CAD build for the part. Positions are in the model's coordinates, mm. Face numbers are marked on the shaded views. A direction names the side the tool comes from. Give positions to 0.01 mm unless a question says otherwise; leave off trailing zeros. Write each loop counter-clockwise with the first axis right and the second up, starting at its lowest first coordinate (ties: lowest second). Pieces come first, ordered by that corner, then holes. Notation, with made-up numbers: M -37.5,-1.75 L -1.5,-1.75 A11 ccw -1.5,2.25 Z; hole C 65,-17.75 d6. An arc over 180 degrees is marked long. One line per question, with ' | ' between items. Start each with the question number.
1. Cut at A-A, the plane x = 7. Write the cut outline in (y, z), then the cut area to 3 significant figures.
2. Wall check: L1, parallel to Y at x = 8.25, z = -1.25; L2, parallel to Z at x = -7, y = 0.4; L3, parallel to Y at x = -0.5, z = -3. Give the ranges that are in metal, low to high.
3. Cut at B-B, the plane y = 1.25. Write the cut outline in (x, z), then the cut area to 3 significant figures.
4. Flat gauge pins, fed straight in: pin 1 (1 mm diameter, centred on y = 5.5, z = 3.5, fed in from +X); pin 2 (5 mm diameter, centred on y = 8, z = -2, fed in from -X); pin 3 (1.5 mm diameter, centred on x = 3, y = 2, fed in from -Z); pin 4 (1.6 mm diameter, centred on x = -7, z = 0, fed in from +Y). Where does each tip first touch, or does it go through?
5. Which spindle directions (+Z, -Z, +X, -X, +Y, -Y) get a long thin tool onto all of the face, cutting with end or side? Do the marked faces 1 and 2. Say none if no direction does.
```python
from build123d import *

# Parameters (mm, degrees)
BOSS_EXTRUDE1_DEPTH = 1
SKETCH2_R           = 5.5
BOSS_EXTRUDE2_DEPTH = 8
FILLET1_R           = 5


with BuildPart() as part:
    # Sketch1 → Boss-Extrude1 (new body)
    with BuildSketch(Plane(origin=(0, 0, 0), x_dir=(1, 0, 0), z_dir=(0, 1, 0))):
        with BuildLine():
            ThreePointArc((-8, 0), (-7, 1), (-6, 0))
            ThreePointArc((-6, 0), (-5.905505906, 1.060660172), (-5.625, 2.087911636))
            ThreePointArc((-5.625, 2.087911636), (-6.926553741, 2.498920897), (-8.25, 2.165063509))
            ThreePointArc((-8.25, 2.165063509), (-9.165063509, 1.25), (-9.5, 0))
            Line((-9.5, 0), (-8, 0))
        make_face()
        with BuildLine():
            ThreePointArc((-5.625, -2.087911636), (-5.905505906, -1.060660172), (-6, 0))
            ThreePointArc((-6, 0), (-7, -1), (-8, 0))
            Line((-8, 0), (-9.5, 0))
            ThreePointArc((-9.5, 0), (-9.165063509, -1.25), (-8.25, -2.165063509))
            ThreePointArc((-8.25, -2.165063509), (-6.926553741, -2.498920897), (-5.625, -2.087911636))
        make_face()
        with BuildLine():
            ThreePointArc((-5.625, 2.087911636), (-5.905505906, 1.060660172), (-6, 0))
            Line((-6, 0), (-4.5, 0))
            ThreePointArc((-4.5, 0), (-4.799147892, 1.185854123), (-5.625, 2.087911636))
        make_face()
        with BuildLine():
            Line((-4.5, 0), (-6, 0))
            ThreePointArc((-6, 0), (-5.905505906, -1.060660172), (-5.625, -2.087911636))
            ThreePointArc((-5.625, -2.087911636), (-4.799147892, -1.185854123), (-4.5, 0))
        make_face()
        with BuildLine():
            ThreePointArc((-8.25, 2.165063509), (-6.926553741, 2.498920897), (-5.625, 2.087911636))
            ThreePointArc((-5.625, 2.087911636), (-4.58398805, 3.871311606), (-3, 5.196152423))
            Line((-3, 5.196152423), (-8.25, 2.165063509))
        make_face()
        with BuildLine():
            ThreePointArc((-3, -5.196152423), (-4.58398805, -3.871311606), (-5.625, -2.087911636))
            ThreePointArc((-5.625, -2.087911636), (-6.926553741, -2.498920897), (-8.25, -2.165063509))
            Line((-8.25, -2.165063509), (-3, -5.196152423))
        make_face()
        with BuildLine():
            Line((4.5, 0), (-4.5, 0))
            ThreePointArc((-4.5, 0), (-4.799147892, -1.185854123), (-5.625, -2.087911636))
            ThreePointArc((-5.625, -2.087911636), (-4.58398805, -3.871311606), (-3, -5.196152423))
            Line((-3, -5.196152423), (3, -5.196152423))
            ThreePointArc((3, -5.196152423), (4.58398805, -3.871311606), (5.625, -2.087911636))
            ThreePointArc((5.625, -2.087911636), (4.799147892, -1.185854123), (4.5, 0))
        make_face()
        with BuildLine():
            ThreePointArc((-5.625, 2.087911636), (-4.799147892, 1.185854123), (-4.5, 0))
            Line((-4.5, 0), (4.5, 0))
            ThreePointArc((4.5, 0), (4.799147892, 1.185854123), (5.625, 2.087911636))
            ThreePointArc((5.625, 2.087911636), (4.58398805, 3.871311606), (3, 5.196152423))
            ThreePointArc((3, 5.196152423), (0, 6), (-3, 5.196152423))
            ThreePointArc((-3, 5.196152423), (-4.58398805, 3.871311606), (-5.625, 2.087911636))
        make_face()
        with BuildLine():
            Line((3, -5.196152423), (-3, -5.196152423))
            ThreePointArc((-3, -5.196152423), (0, -6), (3, -5.196152423))
        make_face()
        with BuildLine():
            ThreePointArc((3, 5.196152423), (4.58398805, 3.871311606), (5.625, 2.087911636))
            ThreePointArc((5.625, 2.087911636), (6.926553741, 2.498920897), (8.25, 2.165063509))
            Line((8.25, 2.165063509), (3, 5.196152423))
        make_face()
        with BuildLine():
            ThreePointArc((8.25, -2.165063509), (6.926553741, -2.498920897), (5.625, -2.087911636))
            ThreePointArc((5.625, -2.087911636), (4.58398805, -3.871311606), (3, -5.196152423))
            Line((3, -5.196152423), (8.25, -2.165063509))
        make_face()
        with BuildLine():
            ThreePointArc((5.625, 2.087911636), (4.799147892, 1.185854123), (4.5, 0))
            Line((4.5, 0), (6, 0))
            ThreePointArc((6, 0), (5.905505906, 1.060660172), (5.625, 2.087911636))
        make_face()
        with BuildLine():
            Line((6, 0), (4.5, 0))
            ThreePointArc((4.5, 0), (4.799147892, -1.185854123), (5.625, -2.087911636))
            ThreePointArc((5.625, -2.087911636), (5.905505906, -1.060660172), (6, 0))
        make_face()
        with BuildLine():
            ThreePointArc((8, 0), (7, -1), (6, 0))
            ThreePointArc((6, 0), (5.905505906, -1.060660172), (5.625, -2.087911636))
            ThreePointArc((5.625, -2.087911636), (6.926553741, -2.498920897), (8.25, -2.165063509))
            Line((8.25, -2.165063509), (8.25, 0))
            Line((8.25, 0), (8, 0))
        make_face()
        with BuildLine():
            ThreePointArc((5.625, 2.087911636), (5.905505906, 1.060660172), (6, 0))
            ThreePointArc((6, 0), (7, 1), (8, 0))
            Line((8, 0), (8.25, 0))
            Line((8.25, 0), (8.25, 2.165063509))
            ThreePointArc((8.25, 2.165063509), (6.926553741, 2.498920897), (5.625, 2.087911636))
        make_face()
        with BuildLine():
            ThreePointArc((9.5, 0), (9.165063509, 1.25), (8.25, 2.165063509))
            Line((8.25, 2.165063509), (8.25, 0))
            Line((8.25, 0), (9.5, 0))
        make_face()
        with BuildLine():
            Line((8.25, 0), (8.25, -2.165063509))
            ThreePointArc((8.25, -2.165063509), (9.165063509, -1.25), (9.5, 0))
            Line((9.5, 0), (8.25, 0))
        make_face()
    extrude(amount=BOSS_EXTRUDE1_DEPTH)

    # Sketch2 → Boss-Extrude2 (add)
    with BuildSketch(Plane(origin=(0, 1, 0), x_dir=(1, 0, 0), z_dir=(0, 1, 0))):
        with Locations(Location((0, 0, 0), (0, 0, 270))):
            Circle(SKETCH2_R)
    extrude(amount=BOSS_EXTRUDE2_DEPTH)

    # Fillet1
    fillet1_edges = [part.edges().sort_by_distance(p)[0] for p in [
        (0, 9, -5.5),
    ]]
    fillet(fillet1_edges, radius=FILLET1_R)


solid = part.part
```
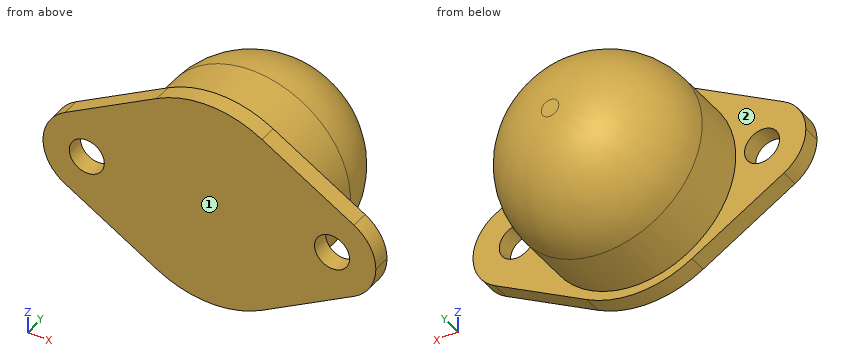
Here are the results:
1) outline: M 0,-2.89 L 1,-2.89 L 1,-1 L 0,-1 Z; M 0,1 L 1,1 L 1,2.89 L 0,2.89 Z | area: 3.77 mm^2
2) L1: 0 to 1 | L2: -2.89 to -1, 1 to 2.89 | L3: 0 to 8.31
3) outline: C 0,0 d11 | area: 95.0 mm^2
4) pin 1: x = 4.37 | pin 2: x = -5.1 | pin 3: z = -5.02 | pin 4: through
5) face 1: +Z, -Z, +X, -X, -Y | face 2: +Y
